Here's how the part is built. I have some questions about the finished solid (model axes, mm). Give positions to 0.01 mm unless a question says otherwise; leave off trailing zeros. Write each loop counter-clockwise with the first axis right and the second up, starting at its lowest first coordinate (ties: lowest second). Pieces come first, ordered by that corner, then holes. Notation, with made-up numbers: (84.5, -16.75) - (142.5, -16.75) arc R28 ccw to (142.5, 21.25) - close; hole circle Ø8 at (71, 31). An arc over 180 degrees is marked (long way). Use a Markdown table: item, result.
```python
from build123d import *

# Parameters (mm, degrees)
F0_W     = 50.8
F0_H     = 101.6
F1_DEPTH = 50.8


with BuildPart() as f1:
    # F0 (on Front) → F1 (new body, symmetric)
    with BuildSketch(Plane.XZ):
        Polygon((-488.5087642836, 0), (-419.1, 74.1955756135), (-50.8, 467.8955756135), (-50.8, 594.8955756135), (-914.4, -319.5044243865), (-787.4, -319.5044243865), align=None)
        Polygon((-177.8, -319.5044243865), (-50.8, -319.5044243865), (-419.1, 74.1955756135), (-488.5087642836, 0), align=None)
        Polygon((-50.8, -421.1044243865), (-50.8, -319.5044243865), (-177.8, -319.5044243865), (-787.4, -319.5044243865), (-914.4, -319.5044243865), (-914.4, -421.1044243865), align=None)
        with BuildLine():
            Line((-50.8, -319.5044243865), (0, -319.5044243865))
            Line((0, -319.5044243865), (0, 499.6455756135))
            ThreePointArc((0, 499.6455756135), (-31.75, 531.3955756135), (0, 563.1455756135))
            Line((0, 563.1455756135), (0, 594.8955756135))
            Line((0, 594.8955756135), (-50.8, 594.8955756135))
            Line((-50.8, 594.8955756135), (-50.8, 467.8955756135))
            Line((-50.8, 467.8955756135), (-50.8, -319.5044243865))
        make_face()
        with BuildLine():
            Line((0, 499.6455756135), (0, -319.5044243865))
            Line((0, -319.5044243865), (50.8, -319.5044243865))
            Line((50.8, -319.5044243865), (50.8, 467.8955756135))
            Line((50.8, 467.8955756135), (50.8, 594.8955756135))
            Line((50.8, 594.8955756135), (0, 594.8955756135))
            Line((0, 594.8955756135), (0, 563.1455756135))
            ThreePointArc((0, 563.1455756135), (22.4506403027, 553.8462159162), (31.75, 531.3955756135))
            ThreePointArc((31.75, 531.3955756135), (22.4506403027, 508.9449353108), (0, 499.6455756135))
        make_face()
        with Locations((25.4, -370.3044243865)):
            Rectangle(F0_W, F0_H)
        with Locations((-25.4, -370.3044243865)):
            Rectangle(F0_W, F0_H)
        Polygon((177.8, -319.5044243865), (50.8, -319.5044243865), (50.8, -421.1044243865), (914.4, -421.1044243865), (914.4, -319.5044243865), (787.4, -319.5044243865), align=None)
        Polygon((50.8, 594.8955756135), (50.8, 467.8955756135), (419.1, 74.1955756135), (488.5087642836, 0), (787.4, -319.5044243865), (914.4, -319.5044243865), align=None)
        Polygon((419.1, 74.1955756135), (50.8, -319.5044243865), (177.8, -319.5044243865), (488.5087642836, 0), align=None)
    extrude(amount=F1_DEPTH, both=True)


solid = f1.part
```
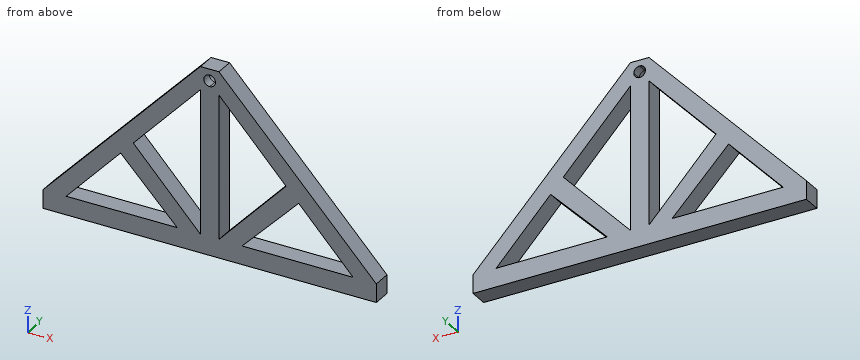
Item 1: If we section it at C-C, the plane z = -204: Write out the boundary of the cut face in (x, y), plus the area to 3 significant figures.
Values:
| item | result |
|---|---|
| outline | (-805.31, -50.8) - (-679.35, -50.8) - (-679.35, 50.8) - (-805.31, 50.8) - close; (-290.12, -50.8) - (-158.85, -50.8) - (-158.85, 50.8) - (-290.12, 50.8) - close; (-50.8, -50.8) - (50.8, -50.8) - (50.8, 50.8) - (-50.8, 50.8) - close; (158.85, -50.8) - (290.12, -50.8) - (290.12, 50.8) - (158.85, 50.8) - close; (679.35, -50.8) - (805.31, -50.8) - (805.31, 50.8) - (679.35, 50.8) - close |
| area | 62,600 mm2 |
Item 2: I need wall thicknesses on line 1 along X through (y, z) = (7, 441); line 2 along X through (y, z) = (-27, -317); line 3 along X through (y, z) = (-4.5, 384). Which ranges of each line are inside material? Lowest first, please. Write a range as [from, to].
Values:
| item | result |
|---|---|
| line 1 | x = [-196.15, -75.96], [-50.8, 50.8], [75.96, 196.15] |
| line 2 | x = [-912.03, -785.06], [-180.24, -53.14], [-50.8, 50.8], [53.14, 180.24], [785.06, 912.03] |
| line 3 | x = [-249.98, -129.28], [-50.8, 50.8], [129.28, 249.98] |
Item 3: If we section it at A-A, the plane x = -250.5: Write out the boundary of the cut face in (y, z).
Values:
| item | result |
|---|---|
| outline | (-50.8, -421.1) - (50.8, -421.1) - (50.8, -319.5) - (-50.8, -319.5) - close; (-50.8, -244.75) - (50.8, -244.75) - (50.8, -106.03) - (-50.8, -106.03) - close; (-50.8, 254.42) - (50.8, 254.42) - (50.8, 383.45) - (-50.8, 383.45) - close |
Item 4: Will these pins go through, and if not, where does the flat tip stop? pin 1 Ø3 at (y, z) = (-17.5, -192) entering from -X; pin 2 Ø12 at (y, z) = (26.5, 87.5) entering from +X; pin 3 Ø6 at (y, z) = (-37, 192.5) entering from +X.
Values:
| item | result |
|---|---|
| pin 1 | stops at x = -795.4 |
| pin 2 | stops at x = 535.67 |
| pin 3 | stops at x = 433.67 |
Item 5: If we section it at D-D, the plane z = 233: Write out the boundary of the cut face in (x, y), plus the area to 3 significant figures.
Values:
| item | result |
|---|---|
| outline | (-392.59, -50.8) - (-270.54, -50.8) - (-270.54, 50.8) - (-392.59, 50.8) - close; (-50.8, -50.8) - (50.8, -50.8) - (50.8, 50.8) - (-50.8, 50.8) - close; (270.54, -50.8) - (392.59, -50.8) - (392.59, 50.8) - (270.54, 50.8) - close |
| area | 35,100 mm2 |
Item 6: If we section it at B-B, the plane y = 29.5: Write out the boundary of the cut face in (x, z), plus the area to 3 significant figures.
Values:
| item | result |
|---|---|
| outline | (-914.4, -421.1) - (914.4, -421.1) - (914.4, -319.5) - (50.8, 594.9) - (-50.8, 594.9) - (-914.4, -319.5) - close; hole (-787.4, -319.5) - (-177.8, -319.5) - (-488.51, 0) - close; hole (-419.1, 74.2) - (-50.8, -319.5) - (-50.8, 467.9) - close; hole circle Ø63.5 at (0, 531.4); hole (50.8, -319.5) - (419.1, 74.2) - (50.8, 467.9) - close; hole (177.8, -319.5) - (787.4, -319.5) - (488.51, 0) - close |
| area | 580,000 mm2 |
